Work out the finished part from the listing and answer in its coordinate system (mm). Face numbers are marked on the shaded views. A direction names the side the tool comes from. Give positions to 0.01 mm unless a question says otherwise; leave off trailing zeros. Write each loop counter-clockwise with the first axis right and the second up, starting at its lowest first coordinate (ties: lowest second). Pieces come first, ordered by that corner, then holes.
1) Straight lines are drawn through the part: probe 1 along Y at (x, z) = (1.8, 18.5); probe 2 along X at (y, z) = (7.5, 4); probe 3 along Z at (x, y) = (8.25, -4). For each, find the intervals that lie inside material, in ascending order.
2) Given pin 1 Ø1.5 at (x, y) = (14.5, -6.5) entering from -Z; pin 2 Ø5.5 at (x, y) = (13.5, 1.5) entering from +Z; pin 3 Ø5 at (x, z) = (15, -20) entering from -Y, each flat-ended and moving along its own axis, determine where each tip first touches the part or whether it passes through.
3) Find section A-A (y = -9.5). Determine the outline of the cut face in (x, z).
4) Find section B-B (z = 18.5). Determine the outline of the cut face in (x, y), plus the area to 3 significant figures.
5) A tool of negligible diameter and unlimited length cuts with its end or side. For the marked faces 1, 2 and 3, from which of +Z, -Z, +X, -X, +Y, -Y can it reach the whole face along a straight path? Write none if from no direction.
6) Find section C-C (x = 2.75). Determine the outline of the cut face in (y, z).
7) Find section D-D (y = -6.25). Determine the outline of the cut face in (x, z).
8) Determine the mould class of the marked faces 4, 5 and 6 for opening direction Y: pulls with the +Y half, pulls with the -Y half, needs draft (parallel to the pull), parting line crosses it, or undercut.
```python
from build123d import *

# Parameters (mm, degrees)
SKETCH1_W           = 45
SKETCH1_H           = 25
BOSS_EXTRUDE1_DEPTH = 5
SKETCH2_R           = 1.5
CUT_EXTRUDE1_DEPTH  = 27.220221204
CUT_EXTRUDE2_DEPTH  = 27.220221204
CHAMFER2_SIZE       = 2
BOSS_EXTRUDE2_START = -10
BOSS_EXTRUDE2_DEPTH = 10
FILLET1_R           = 1


with BuildPart() as part:
    # Sketch1 → Boss-Extrude1 (new body)
    with BuildSketch(Plane(origin=(0, 0, 0), x_dir=(0, 0, -1), z_dir=(1, 0, 0))):
        Rectangle(SKETCH1_W, SKETCH1_H)
    extrude(amount=BOSS_EXTRUDE1_DEPTH)

    # Sketch2 → Cut-Extrude1 (cut, through all)
    with BuildSketch(Plane(origin=(5, 0, 0), x_dir=(0, 0, -1), z_dir=(1, 0, 0))):
        with Locations((-18.5, -9.5)):
            Circle(SKETCH2_R)
        with Locations((18.5, -9.5)):
            Circle(SKETCH2_R)
    extrude(amount=-CUT_EXTRUDE1_DEPTH, mode=Mode.SUBTRACT)

    # Sketch3 → Cut-Extrude2 (cut, through all)
    with BuildSketch(Plane(origin=(5, 0, 0), x_dir=(0, 0, -1), z_dir=(1, 0, 0))):
        Polygon((-12.5, 9.80361421), (-12.5, -5.599476508), (2.5, -5.599476508), align=None)
        Polygon((-2.5, 9.80361421), (12.5, 9.80361421), (12.5, -5.599476508), align=None)
    extrude(amount=-CUT_EXTRUDE2_DEPTH, mode=Mode.SUBTRACT)

    # Chamfer2
    chamfer2_edges = [part.edges().sort_by_distance(p)[0] for p in [
        (0, 0, 22.5),
        (0, 0, -22.5),
    ]]
    chamfer(chamfer2_edges, length=CHAMFER2_SIZE)

    # Sketch4 → Boss-Extrude2 (add)
    with BuildSketch(Plane(origin=(0, 0, -22.5), x_dir=(-1, 0, 0), z_dir=(0, 0, -1)).offset(BOSS_EXTRUDE2_START)):
        Polygon((-5, -5), (-21.490292585, -5), (-5, 11.490292585), align=None)
    extrude(amount=BOSS_EXTRUDE2_DEPTH)

    # Fillet1
    fillet1_edges = [part.edges().sort_by_distance(p)[0] for p in [
        (5, 11.490292585, -17.5),
        (21.490292585, -5, -17.5),
    ]]
    fillet(fillet1_edges, radius=FILLET1_R)


solid = part.part
```
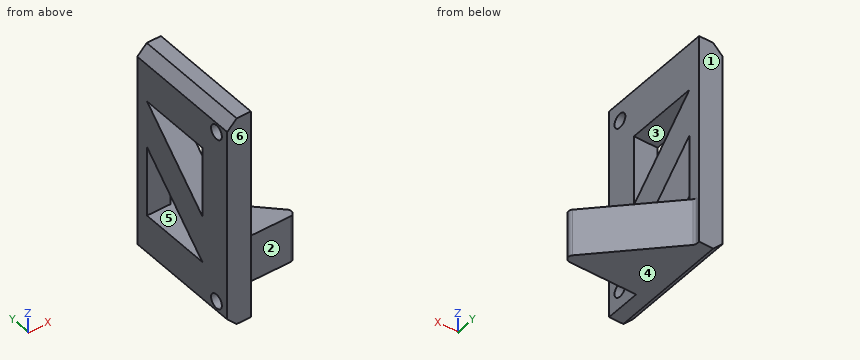
Results:
1. probe 1: y = -12.5 to -11, -8 to 12.5
1. probe 2: x = 0 to 5
1. probe 3: z = -22.5 to -12.5
2. pin 1: passes through
2. pin 2: stops at z = -12.5
2. pin 3: stops at y = -5
3. outline: (0, -20.5) - (2, -22.5) - (5, -22.5) - (5, -20) - (0, -20) - close; (0, -17) - (5, -17) - (5, 17) - (0, 17) - close; (0, 20) - (5, 20) - (5, 22.5) - (2, 22.5) - (0, 20.5) - close
4. outline: (0, -12.5) - (5, -12.5) - (5, -11) - (0, -11) - close; (0, -8) - (5, -8) - (5, 12.5) - (0, 12.5) - close
4. area: 110 mm2
5. face 1: +Z, -Z, +X, -X, +Y
5. face 2: +Z, -Z, +X, -Y
5. face 3: +X, -X
6. outline: (-12.5, -22.5) - (12.5, -22.5) - (12.5, 22.5) - (-12.5, 22.5) - close; hole circle Ø3 at (-9.5, -18.5); hole circle Ø3 at (-9.5, 18.5); hole (-5.6, -12.5) - (9.8, -12.5) - (9.8, 2.5) - close; hole (-5.6, -2.5) - (9.8, 12.5) - (-5.6, 12.5) - close
7. outline: (0, -20.5) - (2, -22.5) - (5, -22.5) - (5, 22.5) - (2, 22.5) - (0, 20.5) - close
8. face 4: needs draft
8. face 5: undercut
8. face 6: pulls with the -Y half
